from build123d import *

# Parameters (mm, degrees)
SKETCH_1_R      = 2.1
SKETCH_1_R_2    = 1.4
EXTRUDE_1_DEPTH = 2
FILLET_1_R      = 1


with BuildPart() as part:
    # 草图1 → 凸台-拉伸1 (new body)
    with BuildSketch(Plane.XY):
        Polygon((87.5, -11), (87.5, -51), (97.5, -51), (97.5, -42), (142.5, -42), (142.5, -20), (97.5, -20), (97.5, -11), align=None)
        with Locations((92.5, -18)):
            Circle(SKETCH_1_R, mode=Mode.SUBTRACT)
        with Locations((92.5, -44)):
            Circle(SKETCH_1_R, mode=Mode.SUBTRACT)
        with Locations((138.5, -39)):
            Circle(SKETCH_1_R_2, mode=Mode.SUBTRACT)
        with Locations((108.5, -39)):
            Circle(SKETCH_1_R_2, mode=Mode.SUBTRACT)
        with Locations(Location((108.5, -23, 0), (0, 0, 180))):
            Circle(SKETCH_1_R_2, mode=Mode.SUBTRACT)
        with Locations(Location((138.5, -23, 0), (0, 0, 180))):
            Circle(SKETCH_1_R_2, mode=Mode.SUBTRACT)
        with BuildLine():
            Line((132.5, -37.5), (114.5, -37.5))
            ThreePointArc((114.5, -37.5), (113.085786438, -36.914213562), (112.5, -35.5))
            Line((112.5, -35.5), (112.5, -26.5))
            ThreePointArc((112.5, -26.5), (113.085786438, -25.085786438), (114.5, -24.5))
            Line((114.5, -24.5), (132.5, -24.5))
            ThreePointArc((132.5, -24.5), (133.914213562, -25.085786438), (134.5, -26.5))
            Line((134.5, -26.5), (134.5, -35.5))
            ThreePointArc((134.5, -35.5), (133.914213562, -36.914213562), (132.5, -37.5))
        make_face(mode=Mode.SUBTRACT)
    extrude(amount=EXTRUDE_1_DEPTH)

    # 圆角1
    fillet_1_edges = [part.edges().sort_by_distance(p)[0] for p in [
        (97.5, -11, 1),
        (97.5, -20, 1),
        (142.5, -20, 1),
        (142.5, -42, 1),
        (97.5, -42, 1),
        (97.5, -51, 1),
        (87.5, -51, 1),
        (87.5, -11, 1),
    ]]
    fillet(fillet_1_edges, radius=FILLET_1_R)


solid = part.part
Could you check a few things on this model? Use its own coordinates, in mm. A direction names the side the tool comes from. Round coordinates to 2 decimals unless told otherwise and drop trailing zeros. Order: outer loops, then holes, each group sorted by start corner. A loop starts at its lowest first (then second) coordinate and runs counter-clockwise, first axis right, second up.
(1) Imagine slicing it at C-C (x = 125). Write out the boundary of the cut face in (y, z), plus the area to 3 significant figures.
Response values:
outline: (-42, 0) - (-37.5, 0) - (-37.5, 2) - (-42, 2) - close; (-24.5, 0) - (-20, 0) - (-20, 2) - (-24.5, 2) - close
area: 18.0 mm2
(2) Imagine slicing it at D-D (z = 0.95). Count the separate pieces of the cut face and the enclosed holes in it, plus the area to 3 significant figures.
Response values:
separate pieces: 1
enclosed holes: 7
area: 1,050 mm2
(3) Imagine slicing it at B-B (x = 138.5). Write out the boundary of the cut face in (y, z).
Response values:
outline: (-42, 0) - (-40.4, 0) - (-40.4, 2) - (-42, 2) - close; (-37.6, 0) - (-24.4, 0) - (-24.4, 2) - (-37.6, 2) - close; (-21.6, 0) - (-20, 0) - (-20, 2) - (-21.6, 2) - close
(4) Imagine slicing it at A-A (y = -23). Write out the boundary of the cut face in (x, z).
Response values:
outline: (87.5, 0) - (107.1, 0) - (107.1, 2) - (87.5, 2) - close; (109.9, 0) - (137.1, 0) - (137.1, 2) - (109.9, 2) - close; (139.9, 0) - (142.5, 0) - (142.5, 2) - (139.9, 2) - close
(5) Please list where these lines run through material, in increasing order: line 1 along Y through (x, z) = (138.5, 1.25); line 2 along Y through (x, z) = (92.5, 1.25); line 3 along X through (y, z) = (-23, 1.55).
Response values:
line 1: y = -42 to -40.4, -37.6 to -24.4, -21.6 to -20
line 2: y = -51 to -46.1, -41.9 to -20.1, -15.9 to -11
line 3: x = 87.5 to 107.1, 109.9 to 137.1, 139.9 to 142.5
(6) If we mould it in two halves opening along Y, with no side actions, what happens to faces 4 (the cylindrical face through (90.4, -17.91, 0.99)), 5 (the flat face through (120, -42, 1)), 6 (the cylindrical face through (107.47, -38.05, 0.99)), 7 (the flat face through (97.5, -16, 1))? For each: released by +Y, released by -Y, zero draft, split by the parting line, or undercut.
Response values:
face 4: undercut
face 5: released by -Y
face 6: undercut
face 7: zero draft
(7) Which directions (+Z, -Z, +X, -X, +Y, -Y) give clear straight access to the entire face, cutting with the end or side of a thin tool? Please do faces 1 (the flat face through (92, -51, 1)), 2 (the flat face through (97.5, -47, 1)), 3 (the flat face through (123, -24.5, 1)).
Response values:
face 1: +Z, -Z, +X, -X, -Y
face 2: +Z, -Z, +X, -Y
face 3: +Z, -Z
(8) I'm going to push flat-ended pins straight in: pin 1 (1 mm diameter, centred on x = 124, z = 1.5, fed in from +Y); pin 2 (6.5 mm diameter, centred on x = 92.5, y = -44, fed in from +Z); pin 3 (1 mm diameter, centred on x = 125.5, z = 1, fed in from -Y); pin 4 (1 mm diameter, centred on y = -15.5, z = 1, fed in from +X). Where does each tip first touch, or does it pass through?
Response values:
pin 1: stops at y = -20
pin 2: stops at z = 2
pin 3: stops at y = -42
pin 4: stops at x = 97.5
